```python
from build123d import *

# Parameters (mm, degrees)
EXTRUDE_1_DEPTH = 2
SKETCH_2_R      = 0.5
EXTRUDE_2_DEPTH = 58
EXTRUDE_3_REACH = 65.509
SKETCH_3_R      = 0.5


with BuildPart() as part:
    # Эскиз1 → Бобышка-Вытянуть1 (new body)
    with BuildSketch(Plane(origin=(0, 0, 0), x_dir=(0, 0, -1), z_dir=(1, 0, 0))):
        Polygon((0, 58), (16.206306346, 58), (24, 2.54498815), (5.89146837, 0), (0, 0), align=None)
    extrude(amount=EXTRUDE_1_DEPTH)

    # Эскиз2 → Бобышка-Вытянуть2 (add)
    with BuildSketch(Plane(origin=(0, 0, 0), x_dir=(1, 0, 0), z_dir=(0, 1, 0))):
        with BuildLine():
            Line((2, 0), (0, 0))
            Line((0, 0), (0, -1))
            ThreePointArc((0, -1), (1, -2), (2, -1))
            Line((2, -1), (2, 0))
        make_face()
        with Locations(Location((1, -1, 0), (0, 0, 270))):
            Circle(SKETCH_2_R, mode=Mode.SUBTRACT)
    extrude(amount=EXTRUDE_2_DEPTH)

    # Бобышка-Вытянуть3: up to this plane
    extrude_3_end = Plane(origin=(2, 58, 0), z_dir=(0, 1, 0))
    # Эскиз3 → Бобышка-Вытянуть3 (add, up to the surface)
    with BuildSketch(Plane(origin=(0, -0.811954382, -0.114112747), x_dir=(1, 0, 0), z_dir=(0, -0.9902680687415703, -0.13917310096006588)), mode=Mode.PRIVATE) as extrude_3_sk1:
        with BuildLine():
            Line((0, -25.120627543), (0, -24.120627543))
            Line((0, -24.120627543), (2, -24.120627543))
            Line((2, -24.120627543), (2, -25.120627543))
            ThreePointArc((2, -25.120627543), (1, -26.120627543), (0, -25.120627543))
        make_face()
        with Locations(Location((1, -25.120627543, 0), (0, 0, 270))):
            Circle(SKETCH_3_R, mode=Mode.SUBTRACT)
    extrude_3_tool1 = split(extrude(extrude_3_sk1.sketch, amount=-EXTRUDE_3_REACH, mode=Mode.PRIVATE), bisect_by=extrude_3_end, keep=Keep.BOTH, mode=Mode.PRIVATE)
    add(extrude_3_tool1.solids().sort_by_distance((1, 2.819398, -25.952527))[0])


solid = part.part
```
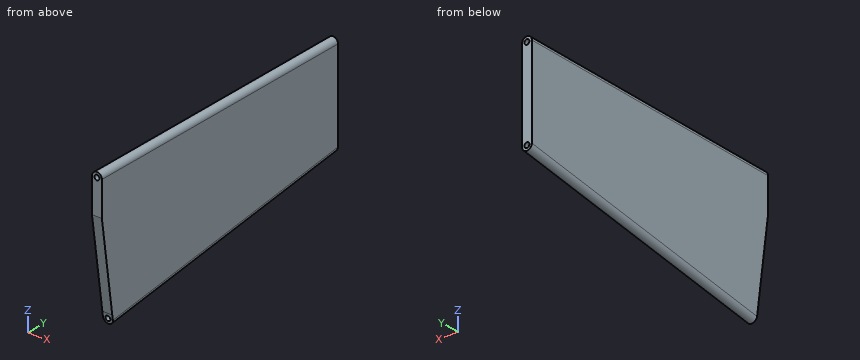
Work out the finished part from the listing and answer in its coordinate system (mm). Coordinates: 2 decimals unless noted, no trailing zeros. Loops run counter-clockwise (first coordinate to the right, second up) from the corner with the lowest first, then second, coordinate; pieces in that order, holes last. Notation, with made-up numbers: M 74,9.25 L 100,9.25 A34 cw 100,42.25 Z; hole C -19.5,62 d5. An arc over 180 degrees is marked long. Use CSV: the item, a comma, the result in double quotes. Start each with the question number.
(1) Consider line 1 (X direction, y = 29, z = 1); line 2 (Z direction, x = 1.25, y = 23.5); line 3 (Z direction, x = 0.6, y = 3.5). Determine where each line is inside the solid, lowest interval first.
(2) Find section B-B, the plane y = 37. State how many separate pieces and enclosed holes the cut face has, then the cut area to 3 significant figures.
(3) Find section A-A, the plane x = 1. Give the vertices of the cut face in (y, z), then the cut area to 3 significant figures.
Recorded:
1,line 1,"x = 0 to 0.5, 1.5 to 2"
1,line 2,"z = -23.04 to -22.5, -21.63 to 0.57, 1.43 to 1.97"
1,line 3,"z = -25.8 to -25.18, -24.57 to 0.7, 1.3 to 1.92"
2,separate pieces,"1"
2,enclosed holes,"2"
2,area,"43.9 mm^2"
3,outline,"M 0,-5.89 L 2.61,-24.5 L 58,-16.71 L 58,0.5 L 0,0.5 Z; M 0,1.5 L 58,1.5 L 58,2 L 0,2 Z; M 2.75,-25.49 L 2.82,-25.98 L 58,-18.23 L 58,-17.72 Z"
3,area,"1,270 mm^2"
